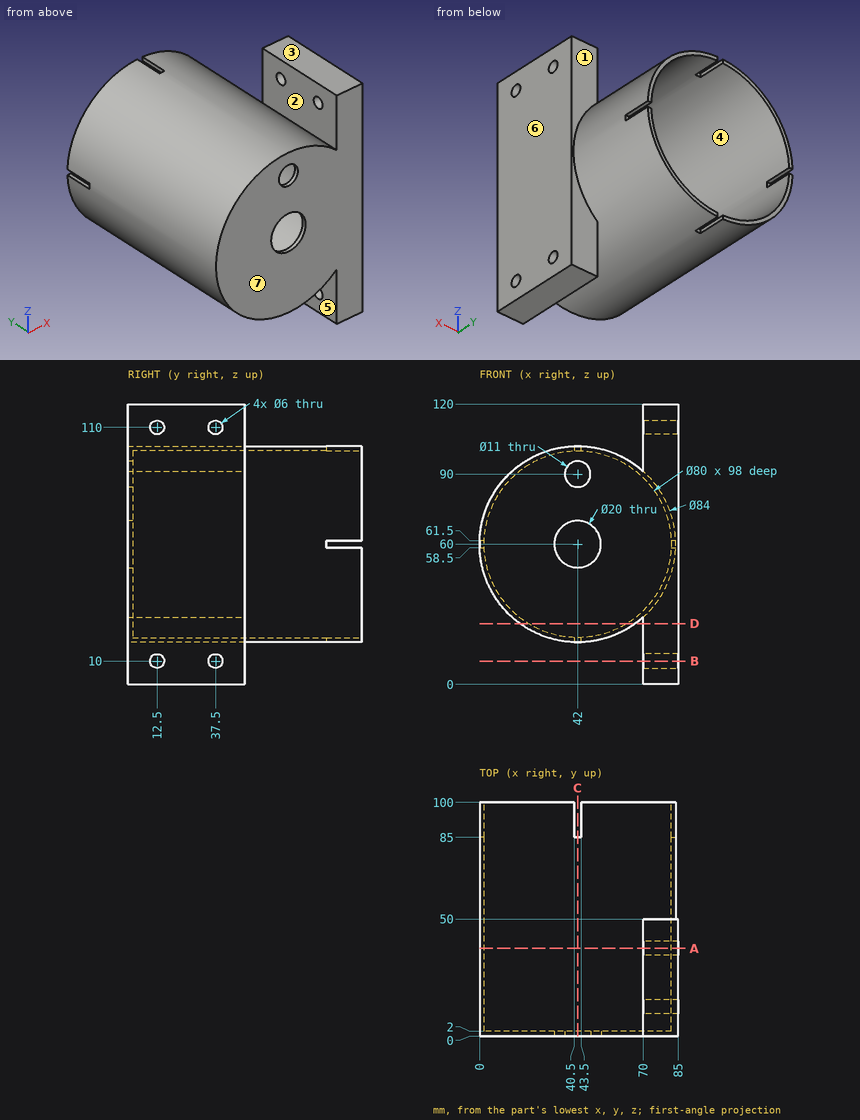
Source: three-view drawing plus pictorial views. Frame: mm from the lowest corner of the part. A direction names the side the tool comes from. Round coordinates to 2 decimals unless told otherwise and drop trailing zeros. Loops run counter-clockwise (first coordinate to the right, second up) from the corner with the lowest first, then second, coordinate; pieces in that order, holes last.
Q1. Section B-B, the plane z = 10. Return loops of the section in (x, y), plus the area to 3 significant figures.
Q2. Ray query, line 1 (Y direction, x = 75, z = 10); line 2 (X direction, y = 38.5, z = 60); line 3 (X direction, y = 1, z = 60). Return the intervals inside material, ascending.
Q3. Access query for the marked faces 1, 2 and 3. Directions: +Z, -Z, +X, -X, +Y, -Y. A direction counts if a zero-diameter tool reaches every point of the face in a straight line with its end or side. Return the directions, or none.
Q4. Section C-C, the plane x = 42. Return loops of the section in (y, z), plus the area to 3 significant figures.
Q5. First-contact query: P1, Ø14.5, axis at y = 33.5, z = 101.5, coming from the -X side; P2, Ø9.5, axis at y = 37.5, z = 10, coming from the -X side; P3, Ø12, axis at y = 50.5, z = 85, coming from the +X side; P4, Ø2, axis at x = 1, z = 60, coming from the +Y side. Flat tips, straight axial feed; report the tip coordinate or a pass-through.
Q6. Section A-A, the plane y = 37.5. Return loops of the section in (x, z).
Q7. Section D-D, the plane z = 26. Return loops of the section in (x, y), plus the area to 3 significant figures.
Q8. Mould query, pull axis X, two halves, no side actions, for the marked faces 4, 5, 6 and 7. Classes: pulls with the +X half, pulls with the -X half, needs draft (parallel to the pull), parting line crosses it, or undercut.
Solutions:
1. outline: (70, 0) - (85, 0) - (85, 9.5) - (70, 9.5) - close; (70, 15.5) - (85, 15.5) - (85, 34.5) - (70, 34.5) - close; (70, 40.5) - (85, 40.5) - (85, 50) - (70, 50) - close
1. area: 570 mm2
2. line 1: y = 0 to 9.5, 15.5 to 34.5, 40.5 to 50
2. line 2: x = 0 to 2, 82 to 85
2. line 3: x = 0 to 32, 52 to 85
3. face 1: +X, +Y
3. face 2: +Z, +Y, -Y
3. face 3: +Z, +X, -X, +Y, -Y
4. outline: (0, 18) - (85, 18) - (85, 20) - (2, 20) - (2, 50) - (0, 50) - close; (0, 70) - (2, 70) - (2, 84.5) - (0, 84.5) - close; (0, 95.5) - (2, 95.5) - (2, 100) - (85, 100) - (85, 102) - (0, 102) - close
4. area: 438 mm2
5. P1: stops at x = 17.69
5. P2: stops at x = 70
5. P3: stops at x = 85
5. P4: stops at y = 85
6. outline: (70, 0) - (85, 0) - (85, 7) - (70, 7) - close; (70, 13) - (85, 13) - (85, 107) - (70, 107) - (70, 91.3) arc R42 ccw (long way) to (70, 28.7) - close; (70, 113) - (85, 113) - (85, 120) - (70, 120) - close; hole circle Ø80 at (42, 60)
7. outline: (17.34, 0) - (66.66, 0) - (66.66, 100) - (63.07, 100) - (63.07, 2) - (20.93, 2) - (20.93, 100) - (17.34, 100) - close; (70, 0) - (85, 0) - (85, 50) - (70, 50) - close
7. area: 1,550 mm2
8. face 4: undercut
8. face 5: undercut
8. face 6: pulls with the +X half
8. face 7: needs draft
